Build history of the part. All positions in model axes, mm. Round coordinates to 2 decimals unless told otherwise and drop trailing zeros. Order: outer loops, then holes, each group sorted by start corner. A loop starts at its lowest first (then second) coordinate and runs counter-clockwise, first axis right, second up. Notation, with made-up numbers: (75, 62) -> (128, 62) arc R19 ccw to (128, 79) -> close; hole circle Ø3 at (60.5, 41.25). An arc over 180 degrees is marked (long way). Write item = value, one per line.
from build123d import *

# Parameters (mm, degrees)
F0_R     = 3.175
F1_DEPTH = 25.4


with BuildPart() as f1:
    # F0 (on Front) → F1 (new body)
    with BuildSketch(Plane.XZ):
        with BuildLine():
            Line((0, 31.75), (0, 19.05))
            ThreePointArc((0, 19.05), (5.579616, 5.579616), (19.05, 0))
            Line((19.05, 0), (361.95, 0))
            ThreePointArc((361.95, 0), (375.420384, 5.579616), (381, 19.05))
            Line((381, 19.05), (381, 31.75))
            ThreePointArc((381, 31.75), (375.420384, 45.220384), (361.95, 50.8))
            Line((361.95, 50.8), (19.05, 50.8))
            ThreePointArc((19.05, 50.8), (5.579616, 45.220384), (0, 31.75))
        make_face()
        with Locations((19.05, 25.4)):
            Circle(F0_R, mode=Mode.SUBTRACT)
        with Locations((190.5, 25.4)):
            Circle(F0_R, mode=Mode.SUBTRACT)
        with Locations((361.95, 25.4)):
            Circle(F0_R, mode=Mode.SUBTRACT)
    extrude(amount=F1_DEPTH)


solid = f1.part
Q1. Cut at A-A, the plane x = 190.5. List the corners of the cut face in (y, z) (3 decimals).
Check values:
outline = (-25.4, 0) -> (0, 0) -> (0, 22.225) -> (-25.4, 22.225) -> close; (-25.4, 28.575) -> (0, 28.575) -> (0, 50.8) -> (-25.4, 50.8) -> close
Q2. Probe probe 1 along Z at (x, y) = (190.5, -6.75) (3 decimals); probe 2 along X at (y, z) = (-8, 27); probe 3 along X at (y, z) = (-9.5, 26.5). List the from-to ranges inside material, lowest first.
Check values:
probe_1 = 0 to 22.225, 28.575 to 50.8
probe_2 = 0 to 16.31, 21.79 to 187.76, 193.24 to 359.21, 364.69 to 381
probe_3 = 0 to 16.07, 22.03 to 187.52, 193.48 to 358.97, 364.93 to 381
Q3. Cut at D-D, the plane z = 6. List the corners of the cut face in (x, y), and give its area (3 significant figures).
Check values:
outline = (5.17, -25.4) -> (375.83, -25.4) -> (375.83, 0) -> (5.17, 0) -> close
area = 9,410 mm²
Q4. Flat gauge pins, fed straight in: pin 1 (4 mm diameter, centred on x = 19.05, z = 25.4, fed in from +Y); pin 2 (1.5 mm diameter, centred on y = -18.5, z = 41.5, fed in from -X). Where does each tip first touch, or does it go through?
Check values:
pin_1 = through
pin_2 = 2.26
Q5. Mould opens along Z. For faces 1 (the face through (5.73, -12.52, 45.37)), 2 (the face through (187.33, -12.52, 25.54)), 3 (the face through (0, -13, 25)) say: released by +Z, released by -Z, zero draft, split by the parting line, or undercut.
Check values:
face_1 = released by +Z
face_2 = undercut
face_3 = zero draft
Q6. Cut at B-B, the plane y = -21.5. List the corners of the cut face in (x, z) (3 decimals).
Check values:
outline = (0, 19.05) arc R19.05 ccw to (19.05, 0) -> (361.95, 0) arc R19.05 ccw to (381, 19.05) -> (381, 31.75) arc R19.05 ccw to (361.95, 50.8) -> (19.05, 50.8) arc R19.05 ccw to (0, 31.75) -> close; hole circle Ø6.35 at (19.05, 25.4); hole circle Ø6.35 at (190.5, 25.4); hole circle Ø6.35 at (361.95, 25.4)
Q7. Cut at C-C, the plane z = 25.4. List the corners of the cut face in (x, y) (3 decimals), and give its area (3 significant figures).
Check values:
outline = (0, -25.4) -> (15.875, -25.4) -> (15.875, 0) -> (0, 0) -> close; (22.225, -25.4) -> (187.325, -25.4) -> (187.325, 0) -> (22.225, 0) -> close; (193.675, -25.4) -> (358.775, -25.4) -> (358.775, 0) -> (193.675, 0) -> close; (365.125, -25.4) -> (381, -25.4) -> (381, 0) -> (365.125, 0) -> close
area = 9,190 mm²
